```python
from build123d import *

# Parameters (mm, degrees)
SKETCH1_R           = 1.7
BOSS_EXTRUDE1_DEPTH = 2
CUT_EXTRUDE7_REACH  = 46.286
SKETCH3_R           = 1.7
SKETCH4_R           = 1.7
CUT_EXTRUDE8_DEPTH  = 45.286002303
SKETCH7_R           = 1.7
CUT_EXTRUDE9_DEPTH  = 45.286002303
CUT_EXTRUDE10_REACH = 46.286
SKETCH8_R           = 1.7


with BuildPart() as part:
    # Sketch1 → Boss-Extrude1 (new body)
    with BuildSketch(Plane.XY):
        with BuildLine():
            Line((-33.5, 25), (33.5, 25))
            ThreePointArc((33.5, 25), (35.621320344, 24.121320344), (36.5, 22))
            Line((36.5, 22), (36.5, -22))
            ThreePointArc((36.5, -22), (35.621320344, -24.121320344), (33.5, -25))
            Line((33.5, -25), (-33.5, -25))
            ThreePointArc((-33.5, -25), (-35.621320344, -24.121320344), (-36.5, -22))
            Line((-36.5, -22), (-36.5, 22))
            ThreePointArc((-36.5, 22), (-35.621320344, 24.121320344), (-33.5, 25))
        make_face()
        with Locations((-32.5, -21.5)):
            Circle(SKETCH1_R, mode=Mode.SUBTRACT)
    extrude(amount=BOSS_EXTRUDE1_DEPTH)

    # Sketch3 → Cut-Extrude7 (cut, up to next)
    with BuildSketch(Plane.XY, mode=Mode.PRIVATE) as cut_extrude7_sk1:
        with Locations((32.5, -21.5)):
            Circle(SKETCH3_R)
    cut_extrude7_tool1 = extrude(cut_extrude7_sk1.sketch, amount=CUT_EXTRUDE7_REACH, mode=Mode.PRIVATE) & part.part
    add(cut_extrude7_tool1.solids().sort_by_distance((32.5, -21.5, 0))[0], mode=Mode.SUBTRACT)

    # Sketch4 → Cut-Extrude8 (cut, through all)
    with BuildSketch(Plane.XY.offset(2)):
        with Locations((-32.5, 21.5)):
            Circle(SKETCH4_R)
    extrude(amount=-CUT_EXTRUDE8_DEPTH, mode=Mode.SUBTRACT)

    # Sketch7 → Cut-Extrude9 (cut, through all)
    with BuildSketch(Plane.XY.offset(2)):
        with Locations((32.5, 21.5)):
            Circle(SKETCH7_R)
    extrude(amount=-CUT_EXTRUDE9_DEPTH, mode=Mode.SUBTRACT)

    # Sketch8 → Cut-Extrude10 (cut, up to next)
    with BuildSketch(Plane(origin=(0, 0, 0), x_dir=(-1, 0, 0), z_dir=(0, 0, -1)), mode=Mode.PRIVATE) as cut_extrude10_sk1:
        with Locations((-29.45, 0)):
            Circle(SKETCH8_R)
    cut_extrude10_tool1 = extrude(cut_extrude10_sk1.sketch, amount=-CUT_EXTRUDE10_REACH, mode=Mode.PRIVATE) & part.part
    # Sketch8 → Cut-Extrude10 (cut, up to next)
    with BuildSketch(Plane(origin=(0, 0, 0), x_dir=(-1, 0, 0), z_dir=(0, 0, -1)), mode=Mode.PRIVATE) as cut_extrude10_sk2:
        with Locations((29.45, 0)):
            Circle(SKETCH8_R)
    cut_extrude10_tool2 = extrude(cut_extrude10_sk2.sketch, amount=-CUT_EXTRUDE10_REACH, mode=Mode.PRIVATE) & part.part
    add(cut_extrude10_tool1.solids().sort_by_distance((29.45, 0, 0))[0], mode=Mode.SUBTRACT)
    add(cut_extrude10_tool2.solids().sort_by_distance((-29.45, 0, 0))[0], mode=Mode.SUBTRACT)


solid = part.part
```
Here's how the part is built. I have some questions about the finished solid (model axes, mm). Give positions to 0.01 mm unless a question says otherwise; leave off trailing zeros. Order: outer loops, then holes, each group sorted by start corner. A loop starts at its lowest first (then second) coordinate and runs counter-clockwise, first axis right, second up. Notation, with made-up numbers: (52.25, -8) -> (73.25, -8) arc R19 ccw to (73.25, -4) -> close; hole circle Ø4 at (-29, 33). An arc over 180 degrees is marked (long way). Use CSV: the item, a comma, the result in double quotes. Start each with the question number.
Item 1: Suppose I cut it at B-B (z = 1.15). List the corners of the cut face in (x, y) for me.
Item 2: If I drill on probe 1 along Y at (x, z) = (32.5, 1.4); probe 2 along X at (y, z) = (20, 1.2); probe 3 along X at (y, z) = (-1, 1.8), over which ranges is the centre line in solid material (lowest first)? Write a range as [from, to].
Item 3: Suppose I cut it at C-C (y = 0). List the corners of the cut face in (x, z) for me.
Item 4: Thinking about a two-plate mould opening in Y: for faces 1 (the cylindrical face through (-30.93, -22.15, 0.99)), 2 (the flat face through (1, 0, 0)), 3 (the cylindrical face through (35.64, -24.1, 0.99)), which applies, pulls with the +Y half, pulls with the -Y half, needs draft (parallel to the pull), parting line crosses it, or undercut?
Item 5: I'm going to push flat-ended pins straight in: P1, Ø3, axis at x = -32.5, y = -21.5, coming from the +Z side; P2, Ø3, axis at x = -8, y = -7, coming from the -Z side. Where does each tip first touch, or does it pass through?
Item 6: Suppose I cut it at A-A (x = -32.5). List the corners of the cut face in (y, z) for me, and give its area (3 significant figures).
Answer block:
1,outline,"(-36.5, -22) arc R3 ccw to (-33.5, -25) -> (33.5, -25) arc R3 ccw to (36.5, -22) -> (36.5, 22) arc R3 ccw to (33.5, 25) -> (-33.5, 25) arc R3 ccw to (-36.5, 22) -> close; hole circle Ø3.4 at (-32.5, -21.5); hole circle Ø3.4 at (-32.5, 21.5); hole circle Ø3.4 at (-29.45, 0); hole circle Ø3.4 at (29.45, 0); hole circle Ø3.4 at (32.5, -21.5); hole circle Ø3.4 at (32.5, 21.5)"
2,probe 1,"y = [-25, -23.2], [-19.8, 19.8], [23.2, 25]"
2,probe 2,"x = [-36.5, -33.3], [-31.7, 31.7], [33.3, 36.5]"
2,probe 3,"x = [-36.5, -30.82], [-28.08, 28.08], [30.82, 36.5]"
3,outline,"(-36.5, 0) -> (-31.15, 0) -> (-31.15, 2) -> (-36.5, 2) -> close; (-27.75, 0) -> (27.75, 0) -> (27.75, 2) -> (-27.75, 2) -> close; (31.15, 0) -> (36.5, 0) -> (36.5, 2) -> (31.15, 2) -> close"
4,face 1,"undercut"
4,face 2,"needs draft"
4,face 3,"pulls with the -Y half"
5,P1,"passes through"
5,P2,"stops at z = 0"
6,outline,"(-25, 0) -> (-23.2, 0) -> (-23.2, 2) -> (-25, 2) -> close; (-19.8, 0) -> (19.8, 0) -> (19.8, 2) -> (-19.8, 2) -> close; (23.2, 0) -> (25, 0) -> (25, 2) -> (23.2, 2) -> close"
6,area,"86.4 mm^2"
